CAD build for the part. Positions are in the model's coordinates, mm. Face numbers are marked on the shaded views. A direction names the side the tool comes from. Coordinates: 2 decimals unless noted, no trailing zeros. Order: outer loops, then holes, each group sorted by start corner. A loop starts at its lowest first (then second) coordinate and runs counter-clockwise, first axis right, second up. Notation, with made-up numbers: (4.5, 61.25) - (29.5, 61.25) arc R24 ccw to (29.5, 89.25) - close; hole circle Ø5 at (71.25, 3). An arc over 180 degrees is marked (long way). Return JSON: item names as keys, results as strings.
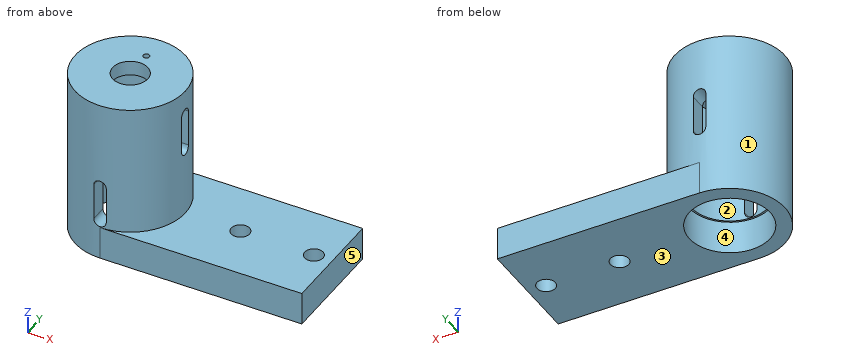
Autodesk Inventor part; units mm, degrees
ref_plane "YZ Plane" through (0, 0, 0) normal (1, 0, 0) x (0, 1, 0)
ref_plane "XZ Plane" through (0, 0, 0) normal (0, 1, 0) x (-1, 0, 0)
ref_plane "XY Plane" through (0, 0, 0) normal (0, 0, 1) x (1, 0, 0)
sketch "Sketch1" plane through (0, 0, 0) normal (0, 0, 1) x (1, 0, 0)
  line L0 (15, 15) -> (70, 15)
  line L1 (70, 15) -> (70, -15)
  line L2 (70, -15) -> (15, -15)
  line L3 (-14, 0) -> (84, 0)
  arc A0 (15, 15) -> (15, -15) centre (15, 0) ccw
  line L4 (0, -21) -> (0, 21)
  line L5 (15, 0) -> (70, 0)
  point P0 (0, 0)
  dimension "d4" = 30
  dimension "d15" = 15
  dimension "d16" = 55
extrude "Extrusion1" add sketch "Sketch1" along normal blind 9
sketch "Sketch2" plane through (0, 0, 9) normal (0, 0, 1) x (1, 0, 0)
  circle A0 centre (15, 0) radius 11
  arc A1 (15, 15) -> (15, -15) centre (15, 0) ccw
  point P0 (0, 0)
  dimension "d7" = 22
extrude "Extrusion2" cut sketch "Sketch2" against normal blind 10
sketch "Sketch3" plane through (0, 0, 9) normal (0, 0, 1) x (1, 0, 0)
  circle A0 centre (45, 0) radius 2.5
  circle A1 centre (65, 0) radius 2.5
  line L0 (70, -15) -> (70, 15)
  point P0 (0, 0)
  dimension "d28" = 3.4
  dimension "d29" = 7
  dimension "d30" = 10
  dimension "d31" = 15
  dimension "d10" = 5
  dimension "d11" = 5
  dimension "d12" = 25
extrude "Extrusion3" cut sketch "Sketch3" against normal blind 25
sketch "Sketch4" plane through (0, 0, 9) normal (0, 0, 1) x (1, 0, 0)
  circle A0 centre (15, 0) radius 15
  circle A1 centre (15, 0) radius 11
  circle A2 centre (15, 0) radius 11
  arc A3 (15, 15) -> (15, -15) centre (15, 0) ccw
  point P0 (0, 0)
extrude "Extrusion4" add sketch "Sketch4" along normal blind 0.001
sketch "Sketch5" plane through (15, 0, 9.001) normal (0, 0, 1) x (1, 0, 0)
  circle A0 centre (0, 0) radius 15
  circle A1 centre (0, 0) radius 10.5
  circle A2 centre (0, 0) radius 15
  point P0 (-15, 0)
  dimension "d19" = 21
extrude "Extrusion5" add sketch "Sketch5" along normal blind 32
sketch "Sketch6" plane through (15, 0, 41.001) normal (0, 0, 1) x (1, 0, 0)
  circle A0 centre (0, 0) radius 4.8
  circle A1 centre (0, 0) radius 15
  circle A2 centre (0, 0) radius 15
  point P0 (-15, 0)
  dimension "d22" = 9.6
extrude "Extrusion6" add sketch "Sketch6" along normal blind 4
sketch "Sketch7" plane through (70, -15, 0) normal (1, 0, 0) x (0, 0, -1)
  line L0 (-45.001, 30) -> (-45.001, 0)
  arc A0 (-38.001, 16.7) -> (-38.001, 13.3) centre (-38.001, 15) ccw
  line L1 (-38.001, 16.7) -> (-28.001, 16.7)
  arc A1 (-28.001, 13.3) -> (-28.001, 16.7) centre (-28.001, 15) ccw
  line L2 (-38.001, 13.3) -> (-28.001, 13.3)
  line L3 (-9, 0) -> (-9, 30)
  line L4 (0, 0) -> (-9, 0)
  point P0 (0, 15)
  dimension "d28" = 3.4
  dimension "d29" = 7
  dimension "d30" = 10
  dimension "d31" = 15
extrude "Extrusion7" cut sketch "Sketch7" against normal blind 50
sketch "Sketch8" plane through (15, 15, 0) normal (0, 1, 0) x (1, 0, 0)
  arc A0 (-1.7, -29.001) -> (1.7, -29.001) centre (0, -29.001) ccw
  arc A1 (1.7, -19.001) -> (-1.7, -19.001) centre (0, -19.001) ccw
  line L0 (-1.7, -29.001) -> (-1.7, -19.001)
  line L1 (1.7, -19.001) -> (1.7, -29.001)
  line L2 (0, -29.001) -> (0, -19.001)
  line L3 (55, -9) -> (0, -9)
  line L4 (55, 0) -> (55, -9)
  line L5 (-15, -45.001) -> (15, -45.001)
  point P0 (-15, 0)
  dimension "d34" = 55
  dimension "d35" = 3.4
  dimension "d36" = 16
  dimension "d37" = 10
extrude "Extrusion8" cut sketch "Sketch8" against normal blind 20
sketch "Sketch9" plane through (15, -15, 0) normal (0, -1, 0) x (1, 0, 0)
  arc A0 (-1.7, 11.001) -> (1.7, 11.001) centre (0, 11.001) ccw
  line L0 (-1.7, 11.001) -> (-1.7, 21.001)
  line L1 (1.7, 11.001) -> (1.7, 21.001)
  arc A1 (1.7, 21.001) -> (-1.7, 21.001) centre (0, 21.001) ccw
  line L2 (15, 45.001) -> (-15, 45.001)
  line L3 (55, 0) -> (55, 9)
  point P0 (-15, 0)
  dimension "d40" = 24
  dimension "d41" = 10
  dimension "d42" = 3.4
  dimension "d43" = 55
extrude "Extrusion9" cut sketch "Sketch9" against normal blind 20
sketch "Sketch10" plane through (15, 0, 45.001) normal (0, 0, 1) x (1, 0, 0)
  circle A0 centre (0, 7.92) radius 0.85
  circle A1 centre (0, 0) radius 15
  line L0 (0, 7.92) -> (0, 0)
  point P0 (-15, 0)
  dimension "d46" = 1.7
  dimension "d47" = 7.92
extrude "Extrusion10" cut sketch "Sketch10" against normal blind 1.8 contours A0
equation "\"d13\" = d12"
properties part number "bearing_mount3"
Item 1: Band-saw the part on B-B, the plane y = 0. Count the separate pieces of the cut face and the enclosed holes in it, then the cut area to 3 significant figures.
Findings below:
{"separate pieces": "5", "enclosed holes": "0", "area": "651 mm²"}
Item 2: Band-saw the part on C-C, the plane y = 13. List the corners of the cut face in (x, z).
Findings below:
{"outline": "(7.52, 0) - (70, 0) - (70, 9) - (22.48, 9) - (22.48, 45) - (7.52, 45) - close; hole (13.3, 19) arc R1.7 ccw to (16.7, 19) - (16.7, 29) arc R1.7 ccw to (13.3, 29) - close"}
Item 3: Mould opens along Y. For the marked faces 1, 2 and 3 say: released by +Y, released by -Y, zero draft, split by the parting line, or undercut.
Findings below:
{"face 1": "split by the parting line", "face 2": "undercut", "face 3": "zero draft"}
Item 4: Drop flat-ended pins along their axis: P1, Ø1.4, axis at x = 15, y = 7.92, coming from the -Z side; P2, Ø2, axis at x = 28, y = -1.5, coming from the -Z side; P3, Ø6, axis at x = 39.5, y = 8.5, coming from the +Z side; P4, Ø1.5, axis at y = -9.5, z = 20.5, coming from the +X side. Give the stop position or say it passes through.
Findings below:
{"P1": "stops at z = 41", "P2": "stops at z = 0", "P3": "stops at z = 9", "P4": "stops at x = 27.18"}
Item 5: Which spindle directions (+Z, -Z, +X, -X, +Y, -Y) get a long thin tool onto all of the face, cutting with end or side? Do the marked faces 4 and 5. Say none if no direction does.
Findings below:
{"face 4": "-Z", "face 5": "+Z, -Z, +X, +Y, -Y"}
Item 6: Band-saw the part on D-D, the plane z = 25. List the corners of the cut face in (x, y), then the cut area to 3 significant figures.
Findings below:
{"outline": "(13.3, 10.36) - (13.3, 14.9) arc R15 ccw (long way) to (16.7, 14.9) - (16.7, 10.36) arc R10.5 cw (long way) to start", "area": "345 mm²"}
Item 7: Wall check: L1, parallel to Y at x = 15, z = 44; L2, parallel to Y at x = 15, z = 42; L3, parallel to Y at x = 15, z = 4.5. Give the ranges that are in metal, low to high. Write a range as [from, to].
Findings below:
{"L1": "y = [-15, -4.8], [4.8, 7.07], [8.77, 15]", "L2": "y = [-15, -4.8], [4.8, 15]", "L3": "y = [-15, -11], [11, 15]"}
Item 8: Band-saw the part on A-A, the plane x = 45. List the corners of the cut face in (y, z), then the cut area to 3 significant figures.
Findings below:
{"outline": "(-15, 0) - (-2.5, 0) - (-2.5, 9) - (-15, 9) - close; (2.5, 0) - (15, 0) - (15, 9) - (2.5, 9) - close", "area": "225 mm²"}
